Model file for the job. Use its own axes, mm. Round coordinates to 2 decimals unless told otherwise and drop trailing zeros. Order: outer loops, then holes, each group sorted by start corner. A loop starts at its lowest first (then second) coordinate and runs counter-clockwise, first axis right, second up. Notation, with made-up numbers: (40, 2) -> (67, 2) arc R23 ccw to (67, 26) -> close; hole circle Ø4 at (71.25, 25.25). An arc over 180 degrees is marked (long way). Use CSV: the item, a comma, the result in double quotes.
Autodesk Inventor part; units mm, degrees
ref_plane "Płaszczyzna konstrukcyjna1" through (-3, -53.7409, -15) normal (0, 0, -1) x (0, 1, 0)
ref_plane "YZ Plane" through (0, 0, 0) normal (1, 0, 0) x (0, 1, 0)
ref_plane "XZ Plane" through (0, 0, 0) normal (0, 1, 0) x (-1, 0, 0)
sketch "Szkic1" plane through (0, 0, 0) normal (0, 0, 1) x (1, 0, 0)
  arc A0 (3, 14.9136) -> (3, 9.2591) centre (3.6454, 12.0864) ccw
  circle A1 centre (3.6454, 12.0864) radius 2.9
  line L0 (4.6454, 14.8085) -> (4.6454, 17.9136)
  line L1 (3, 17.9136) -> (0, 17.9136)
  line L2 (4.6454, 17.9136) -> (11.6454, 17.9136)
  line L3 (14.6454, 14.9136) -> (14.6454, -17.9136)
  line L4 (-2.916, -17.9136) -> (18.8782, -17.9136) construction
  line L5 (4.6454, 9.3642) -> (4.6454, -17.9136)
  line L6 (4.6454, -17.9136) -> (14.6454, -17.9136)
  line L7 (11.6454, 17.9136) -> (14.6454, 14.9136)
  point P0 (0, 0)
  dimension "d0" = 45
  dimension "d1" = 3
  dimension "d8" = 30
  dimension "d9" = 1
  dimension "d10" = 5.8
  dimension "d11" = 11
ref_plane "Płaszczyzna konstrukcyjna1" through (-3, -53.7409, -15) normal (0, 0, -1) x (0, 1, 0)
extrude "Wyciągnięcie proste1" add sketch "Szkic1" against normal up to surface (15 mm away) contours L0 L2 L7 L3 L6 L5 A1
mirror "Odbij1" about plane through (14.6454, -17.9136, 0) normal (0, -1, 0) of "Wyciągnięcie proste1"
sketch "Szkic2" plane through (14.6454, 14.9136, 0) normal (1, 0, 0) x (0, 0, -1)
  circle A0 centre (7.5, -10.4312) radius 2.1 construction
  circle A1 centre (7.5, -32.8273) radius 3.25 construction
  circle A2 centre (7.5, -55.2233) radius 2.1 construction
  circle A3 centre (7.5, -10.4312) radius 1.975
  circle A4 centre (7.5, -55.2233) radius 1.975
  circle A5 centre (7.5, -32.8273) radius 3.25
  circle A6 centre (7.5, -28.9673) radius 2.25
  circle A7 centre (7.5, -42.4703) radius 2.25
  line L0 (7.5, -28.9673) -> (7.5, -36.6873) construction
  line L1 (15, 0) -> (15, -65.6545) construction
  point P0 (0, -14.9136)
  dimension "d5" = 3.95
  dimension "d12" = 4.5
  dimension "d13" = 4.5
  dimension "d14" = 13.503
  dimension "d15" = 9.643
extrude "Wyciągnięcie proste2" cut sketch "Szkic2" against normal through all
properties part number "6xMounting_base"
Q1. Probe line 1 along Y through (x, z) = (7, -7.5); line 2 along Y through (x, z) = (13.5, -9); line 3 along Y through (x, z) = (5.75, -5). List the from-to ranges inside material, lowest first.
From the geometry:
line 1,"y = -53.74 to -42.28, -38.33 to -29.81, -25.31 to -21.16, -11.8 to 2.51, 6.46 to 17.91"
line 2,"y = -51.89 to -41.59, -39.02 to -29.23, -25.88 to -20.8, -12.38 to 3.2, 5.77 to 16.06"
line 3,"y = -53.74 to -49.91, -45.92 to -19.99, -15.84 to 10.09, 14.08 to 17.91"
Q2. Cut at A-A (z = -7.25). Give the cut face in (x, y), plus the area to 3 significant figures.
From the geometry:
outline,"(4.65, -53.74) -> (11.65, -53.74) -> (14.65, -50.74) -> (14.65, -42.27) -> (4.65, -42.27) -> (4.65, -45.19) arc R2.9 cw to (4.65, -50.64) -> close; (4.65, -38.35) -> (14.65, -38.35) -> (14.65, -29.79) -> (4.65, -29.79) -> close; (4.65, -25.32) -> (14.65, -25.32) -> (14.65, -21.15) -> (4.65, -21.15) -> close; (4.65, -11.82) -> (14.65, -11.82) -> (14.65, 2.52) -> (4.65, 2.52) -> close; (4.65, 6.44) -> (14.65, 6.44) -> (14.65, 14.91) -> (11.65, 17.91) -> (4.65, 17.91) -> (4.65, 14.81) arc R2.9 cw to (4.65, 9.36) -> close"
area,"476 mm²"
Q3. Mould opens along Y. For faces 1 (the cylindrical face through (9.715, -41.066, -9.324)), 2 (the flat face through (4.645, -18, -11)), 3 (the flat face through (13.124, 16.435, -7.395)) say: +Y half, -Y half, draft (parallel to the pull), parting line (faces both ways), or undercut.
From the geometry:
face 1,"undercut"
face 2,"draft"
face 3,"+Y half"
Q4. Cut at C-C (y = 13.5). Give the cut face in (x, z).
From the geometry:
outline,"(6.18, -15) -> (14.65, -15) -> (14.65, 0) -> (6.18, 0) -> close"
Q5. Cut at B-B (x = 8.5). Give the cut face in (y, z) (3 decimals), plus the area to 3 significant figures.
From the geometry:
outline,"(-53.741, -15) -> (17.914, -15) -> (17.914, 0) -> (-53.741, 0) -> close; hole circle Ø3.95 at (-40.31, -7.5); hole circle Ø4.5 at (-27.557, -7.5); hole (-15.271, -9.392) arc R2.25 ccw (long way) to (-15.271, -5.608) arc R3.25 ccw (long way) to start; hole circle Ø3.95 at (4.482, -7.5)"
area,"990 mm²"
